Design review of the part built by this model. Coordinates are the model's own, in mm. Coordinates: 2 decimals unless noted, no trailing zeros.
Q1. To check wall thickness, follow probe 1 along Y at (x, z) = (-17.5, 245); probe 2 along Y at (x, z) = (10, 144); probe 3 along X at (y, z) = (-6, 207). State the ranges of each line that lie inside material, in increasing order.
Q2. Add section A-A, the plane z = 242.5. Give the number of separate pieces and of enclosed holes in the cut face, plus the area to 3 significant figures.
Q3. Clearance check with flat-ended pins moving along their axes: pin 1 Ø1.5 at (y, z) = (-14.5, 445) entering from +X; pin 2 Ø8 at (x, z) = (2, 343) entering from -Y; pin 3 Ø4 at (x, z) = (-7, 373) entering from +Y; pin 4 Ø2 at (y, z) = (-14, 274) entering from -X. State where each tip first meets the part, or that it passes through.
from build123d import *

# Parameters (mm, degrees)
SKETCH1_R           = 3.3274
BOSS_EXTRUDE1_DEPTH = 600


with BuildPart() as part:
    # Sketch1 → Boss-Extrude1 (new body)
    with BuildSketch(Plane.XY):
        with BuildLine():
            Line((-13.26278249, 12.048382599), (-9.466223312, 8.222017216))
            ThreePointArc((-9.466223312, 8.222017216), (-7.839336885, 7.128051946), (-5.916892336, 6.7437))
            Line((-5.916892336, 6.7437), (-0.938351009, 6.7437))
            ThreePointArc((-0.938351009, 6.7437), (0.975066153, 7.124302337), (2.597182897, 8.208166094))
            Line((2.597182897, 8.208166094), (6.436676974, 12.047660172))
            ThreePointArc((6.436676974, 12.047660172), (6.761836101, 12.534295195), (6.876016803, 13.108320344))
            Line((6.876016803, 13.108320344), (6.876016803, 14.986))
            ThreePointArc((6.876016803, 14.986), (6.583123584, 15.693106781), (5.876016803, 15.986))
            Line((5.876016803, 15.986), (3.390016803, 15.986))
            Line((3.390016803, 15.986), (3.390016803, 14.986))
            ThreePointArc((3.390016803, 14.986), (0.690016803, 17.018), (3.390016803, 19.05))
            Line((3.390016803, 19.05), (4.390016803, 19.05))
            ThreePointArc((4.390016803, 19.05), (4.972748366, 18.467268437), (5.555479929, 19.05))
            Line((5.555479929, 19.05), (10.055479929, 19.05))
            ThreePointArc((10.055479929, 19.05), (10.648750347, 18.456729582), (11.242020765, 19.05))
            Line((11.242020765, 19.05), (13.081716803, 19.05))
            ThreePointArc((13.081716803, 19.05), (14.849483756, 18.317766953), (15.581716803, 16.55))
            Line((15.581716803, 16.55), (15.581716803, 14.701887799))
            ThreePointArc((15.581716803, 14.701887799), (14.98781258, 14.107983576), (15.581716803, 13.514079353))
            Line((15.581716803, 13.514079353), (15.581716803, 9.000407261))
            ThreePointArc((15.581716803, 9.000407261), (14.977014321, 8.39570478), (15.581716803, 7.791002299))
            Line((15.581716803, 7.791002299), (15.581716803, 6.801))
            ThreePointArc((15.581716803, 6.801), (13.549716803, 4.101), (11.517716803, 6.801))
            Line((11.517716803, 6.801), (12.517716803, 6.801))
            Line((12.517716803, 6.801), (12.517716803, 9.287))
            ThreePointArc((12.517716803, 9.287), (12.224823584, 9.994106781), (11.517716803, 10.287))
            Line((11.517716803, 10.287), (9.640037146, 10.287))
            ThreePointArc((9.640037146, 10.287), (9.066011998, 10.172819299), (8.579376974, 9.847660172))
            Line((8.579376974, 9.847660172), (3.275416803, 4.5437))
            Line((3.275416803, 4.5437), (3.275416803, -2.472632188))
            ThreePointArc((3.275416803, -2.472632188), (3.65601914, -4.38604935), (4.739882897, -6.008166094))
            Line((4.739882897, -6.008166094), (8.579376974, -9.847660172))
            ThreePointArc((8.579376974, -9.847660172), (9.066011998, -10.172819299), (9.640037146, -10.287))
            Line((9.640037146, -10.287), (11.517716803, -10.287))
            ThreePointArc((11.517716803, -10.287), (12.224823584, -9.994106781), (12.517716803, -9.287))
            Line((12.517716803, -9.287), (12.517716803, -6.801))
            Line((12.517716803, -6.801), (11.517716803, -6.801))
            ThreePointArc((11.517716803, -6.801), (13.549716803, -4.101), (15.581716803, -6.801))
            Line((15.581716803, -6.801), (15.581716803, -7.784900507))
            ThreePointArc((15.581716803, -7.784900507), (14.976944942, -8.389672368), (15.581716803, -8.994444229))
            Line((15.581716803, -8.994444229), (15.581716803, -13.530233187))
            ThreePointArc((15.581716803, -13.530233187), (14.961825645, -14.150124345), (15.581716803, -14.770015502))
            Line((15.581716803, -14.770015502), (15.581716803, -16.55))
            ThreePointArc((15.581716803, -16.55), (14.849483756, -18.317766953), (13.081716803, -19.05))
            Line((13.081716803, -19.05), (11.242020765, -19.05))
            ThreePointArc((11.242020765, -19.05), (10.648750347, -18.456729582), (10.055479929, -19.05))
            Line((10.055479929, -19.05), (5.555479929, -19.05))
            ThreePointArc((5.555479929, -19.05), (4.944098366, -18.438618437), (4.332716803, -19.05))
            Line((4.332716803, -19.05), (3.332716803, -19.05))
            ThreePointArc((3.332716803, -19.05), (0.632716803, -17.018), (3.332716803, -14.986))
            Line((3.332716803, -14.986), (3.332716803, -15.986))
            Line((3.332716803, -15.986), (5.818716803, -15.986))
            ThreePointArc((5.818716803, -15.986), (6.525823584, -15.693106781), (6.818716803, -14.986))
            Line((6.818716803, -14.986), (6.818716803, -13.108320344))
            ThreePointArc((6.818716803, -13.108320344), (6.704536101, -12.534295195), (6.379376974, -12.047660172))
            Line((6.379376974, -12.047660172), (2.539882897, -8.208166094))
            ThreePointArc((2.539882897, -8.208166094), (0.917766153, -7.124302337), (-0.995651009, -6.7437))
            Line((-0.995651009, -6.7437), (-5.974192336, -6.7437))
            ThreePointArc((-5.974192336, -6.7437), (-7.896636885, -7.128051946), (-9.523523312, -8.222017216))
            Line((-9.523523312, -8.222017216), (-13.32008249, -12.048382599))
            ThreePointArc((-13.32008249, -12.048382599), (-13.642222082, -12.533572695), (-13.755283197, -13.104887434))
            Line((-13.755283197, -13.104887434), (-13.755283197, -14.986))
            ThreePointArc((-13.755283197, -14.986), (-13.462389979, -15.693106781), (-12.755283197, -15.986))
            Line((-12.755283197, -15.986), (-10.269283197, -15.986))
            Line((-10.269283197, -15.986), (-10.269283197, -14.986))
            ThreePointArc((-10.269283197, -14.986), (-7.569283197, -17.018), (-10.269283197, -19.05))
            Line((-10.269283197, -19.05), (-11.315016833, -19.05))
            ThreePointArc((-11.315016833, -19.05), (-11.921258393, -18.44375844), (-12.527499953, -19.05))
            Line((-12.527499953, -19.05), (-16.98793888, -19.05))
            ThreePointArc((-16.98793888, -19.05), (-17.564834103, -18.473104777), (-18.141729326, -19.05))
            Line((-18.141729326, -19.05), (-20.018283197, -19.05))
            ThreePointArc((-20.018283197, -19.05), (-21.78605015, -18.317766953), (-22.518283197, -16.55))
            Line((-22.518283197, -16.55), (-22.518283197, -14.770015502))
            ThreePointArc((-22.518283197, -14.770015502), (-21.89839204, -14.150124345), (-22.518283197, -13.530233187))
            Line((-22.518283197, -13.530233187), (-22.518283197, -8.994444229))
            ThreePointArc((-22.518283197, -8.994444229), (-21.913511336, -8.389672368), (-22.518283197, -7.784900507))
            Line((-22.518283197, -7.784900507), (-22.518283197, -6.801))
            ThreePointArc((-22.518283197, -6.801), (-20.486283197, -4.101), (-18.454283197, -6.801))
            Line((-18.454283197, -6.801), (-19.454283197, -6.801))
            Line((-19.454283197, -6.801), (-19.454283197, -9.287))
            ThreePointArc((-19.454283197, -9.287), (-19.161389979, -9.994106781), (-18.454283197, -10.287))
            Line((-18.454283197, -10.287), (-15.690222352, -10.287))
            ThreePointArc((-15.690222352, -10.287), (-15.116197203, -10.172819299), (-14.62956218, -9.847660172))
            Line((-14.62956218, -9.847660172), (-10.790068102, -6.008166094))
            ThreePointArc((-10.790068102, -6.008166094), (-9.706204346, -4.38604935), (-9.325602008, -2.472632188))
            Line((-9.325602008, -2.472632188), (-9.325602008, 2.472632188))
            ThreePointArc((-9.325602008, 2.472632188), (-9.706204346, 4.38604935), (-10.790068102, 6.008166094))
            Line((-10.790068102, 6.008166094), (-14.62956218, 9.847660172))
            ThreePointArc((-14.62956218, 9.847660172), (-15.116197203, 10.172819299), (-15.690222352, 10.287))
            Line((-15.690222352, 10.287), (-18.470283197, 10.287))
            ThreePointArc((-18.470283197, 10.287), (-19.177389979, 9.994106781), (-19.470283197, 9.287))
            Line((-19.470283197, 9.287), (-19.470283197, 6.801))
            Line((-19.470283197, 6.801), (-18.454283197, 6.801))
            ThreePointArc((-18.454283197, 6.801), (-20.486283197, 4.101), (-22.518283197, 6.801))
            Line((-22.518283197, 6.801), (-22.518283197, 7.791002299))
            ThreePointArc((-22.518283197, 7.791002299), (-21.913580716, 8.39570478), (-22.518283197, 9.000407261))
            Line((-22.518283197, 9.000407261), (-22.518283197, 13.514079353))
            ThreePointArc((-22.518283197, 13.514079353), (-21.924378975, 14.107983576), (-22.518283197, 14.701887799))
            Line((-22.518283197, 14.701887799), (-22.518283197, 16.55))
            ThreePointArc((-22.518283197, 16.55), (-21.78605015, 18.317766953), (-20.018283197, 19.05))
            Line((-20.018283197, 19.05), (-18.058059148, 19.05))
            ThreePointArc((-18.058059148, 19.05), (-17.472421173, 18.464362025), (-16.886783197, 19.05))
            Line((-16.886783197, 19.05), (-12.338361419, 19.05))
            ThreePointArc((-12.338361419, 19.05), (-11.7540173, 18.465655881), (-11.169673181, 19.05))
            Line((-11.169673181, 19.05), (-10.211983197, 19.05))
            ThreePointArc((-10.211983197, 19.05), (-7.511983197, 17.018), (-10.211983197, 14.986))
            Line((-10.211983197, 14.986), (-10.211983197, 15.986))
            Line((-10.211983197, 15.986), (-12.697983197, 15.986))
            ThreePointArc((-12.697983197, 15.986), (-13.405089979, 15.693106781), (-13.697983197, 14.986))
            Line((-13.697983197, 14.986), (-13.697983197, 13.104887434))
            ThreePointArc((-13.697983197, 13.104887434), (-13.584922082, 12.533572695), (-13.26278249, 12.048382599))
        make_face()
        with Locations((-3.468283197, 0)):
            Circle(SKETCH1_R, mode=Mode.SUBTRACT)
        with BuildLine():
            Line((14.158897896, 12.521284057), (14.158897896, 14.421284057))
            ThreePointArc((14.158897896, 14.421284057), (13.426664849, 16.189051009), (11.658897896, 16.921284057))
            Line((11.658897896, 16.921284057), (9.758897896, 16.921284057))
            Line((9.758897896, 16.921284057), (9.758897896, 12.521284057))
            Line((9.758897896, 12.521284057), (14.158897896, 12.521284057))
        make_face(mode=Mode.SUBTRACT)
        with BuildLine():
            Line((-15.841102104, 12.521284057), (-20.241102104, 12.521284057))
            Line((-20.241102104, 12.521284057), (-20.241102104, 14.421284057))
            ThreePointArc((-20.241102104, 14.421284057), (-19.508869057, 16.189051009), (-17.741102104, 16.921284057))
            Line((-17.741102104, 16.921284057), (-15.841102104, 16.921284057))
            Line((-15.841102104, 16.921284057), (-15.841102104, 12.521284057))
        make_face(mode=Mode.SUBTRACT)
        with BuildLine():
            Line((-15.841102104, -17.478715943), (-15.841102104, -13.078715943))
            Line((-15.841102104, -13.078715943), (-20.241102104, -13.078715943))
            Line((-20.241102104, -13.078715943), (-20.241102104, -14.978715943))
            ThreePointArc((-20.241102104, -14.978715943), (-19.508869057, -16.746482896), (-17.741102104, -17.478715943))
            Line((-17.741102104, -17.478715943), (-15.841102104, -17.478715943))
        make_face(mode=Mode.SUBTRACT)
        with BuildLine():
            Line((14.158897896, -14.978715943), (14.158897896, -13.078715943))
            Line((14.158897896, -13.078715943), (9.758897896, -13.078715943))
            Line((9.758897896, -13.078715943), (9.758897896, -17.478715943))
            Line((9.758897896, -17.478715943), (11.658897896, -17.478715943))
            ThreePointArc((11.658897896, -17.478715943), (13.426664849, -16.746482896), (14.158897896, -14.978715943))
        make_face(mode=Mode.SUBTRACT)
    extrude(amount=BOSS_EXTRUDE1_DEPTH)


solid = part.part
Here are the results:
1. probe 1: y = -18.48 to -17.48, -13.08 to -10.29, 10.29 to 12.52, 16.92 to 18.47
1. probe 2: y = -19.05 to -17.48, -13.08 to -10.29, 10.29 to 12.52, 16.92 to 19.05
1. probe 3: x = -22.59 to -18.38, -10.78 to 4.73, 11.45 to 15.65
2. separate pieces: 1
2. enclosed holes: 5
2. area: 598 mm2
3. pin 1: stops at x = 15.58
3. pin 2: stops at y = -19.13
3. pin 3: stops at y = 19.04
3. pin 4: stops at x = -22.52
